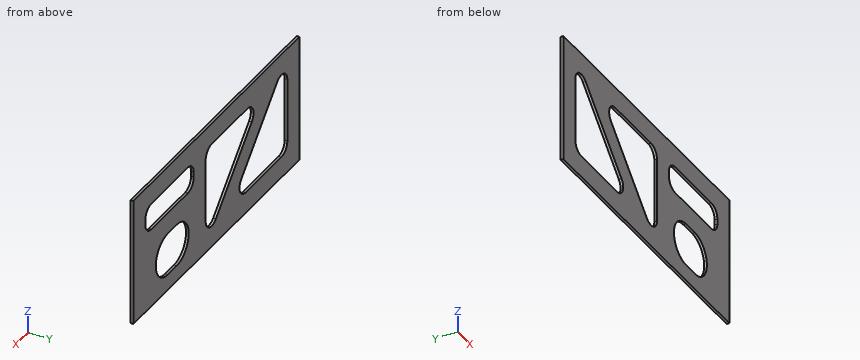
```python
from build123d import *

# Parameters (mm, degrees)
SKETCH1_W           = 352.425
SKETCH1_H           = 152.4
BOSS_EXTRUDE1_DEPTH = 1.5875
CUT_EXTRUDE1_DEPTH  = 4.175


with BuildPart() as part:
    # Sketch1 → Boss-Extrude1 (new body, symmetric)
    with BuildSketch(Plane(origin=(0, 0, 0), x_dir=(1, 0, 0), z_dir=(0, 1, 0))):
        Rectangle(SKETCH1_W, SKETCH1_H)
    extrude(amount=BOSS_EXTRUDE1_DEPTH, both=True)

    # Sketch2 → Cut-Extrude1 (cut, through all)
    with BuildSketch(Plane(origin=(0, 1.5875, 0), x_dir=(1, 0, 0), z_dir=(0, 1, 0))):
        with BuildLine():
            Line((103.1875, 6.35), (84.1375, 6.35))
            ThreePointArc((84.1375, 6.35), (58.7375, 31.75), (84.1375, 57.15))
            Line((84.1375, 57.15), (103.1875, 57.15))
            ThreePointArc((103.1875, 57.15), (128.5875, 31.75), (103.1875, 6.35))
        make_face()
        with BuildLine():
            Line((-138.1125, 50.8), (-61.9125, 50.8))
            ThreePointArc((-61.9125, 50.8), (-50.179229937, 42.960079591), (-52.932243879, 29.119743879))
            Line((-52.932243879, 29.119743879), (-129.132243879, -47.080256121))
            ThreePointArc((-129.132243879, -47.080256121), (-142.972579591, -49.833270063), (-150.8125, -38.1))
            Line((-150.8125, -38.1), (-150.8125, 38.1))
            ThreePointArc((-150.8125, 38.1), (-147.092756121, 47.080256121), (-138.1125, 50.8))
        make_face()
        with BuildLine():
            Line((-66.270451031, -50.8), (9.929548969, -50.8))
            ThreePointArc((9.929548969, -50.8), (18.90980509, -47.080256121), (22.629548969, -38.1))
            Line((22.629548969, -38.1), (22.629548969, 38.1))
            ThreePointArc((22.629548969, 38.1), (14.78962856, 49.833270063), (0.949292847, 47.080256121))
            Line((0.949292847, 47.080256121), (-75.250707153, -29.119743879))
            ThreePointArc((-75.250707153, -29.119743879), (-78.003721094, -42.960079591), (-66.270451031, -50.8))
        make_face()
        with BuildLine():
            Line((60.729548969, -50.8), (138.1125, -50.8))
            ThreePointArc((138.1125, -50.8), (147.092756121, -47.080256121), (150.8125, -38.1))
            Line((150.8125, -38.1), (150.8125, -31.75))
            ThreePointArc((150.8125, -31.75), (147.092756121, -22.769743879), (138.1125, -19.05))
            Line((138.1125, -19.05), (60.729548969, -19.05))
            ThreePointArc((60.729548969, -19.05), (51.749292847, -22.769743879), (48.029548969, -31.75))
            Line((48.029548969, -31.75), (48.029548969, -38.1))
            ThreePointArc((48.029548969, -38.1), (51.749292847, -47.080256121), (60.729548969, -50.8))
        make_face()
    extrude(amount=-CUT_EXTRUDE1_DEPTH, mode=Mode.SUBTRACT)


solid = part.part
```
The model under review builds one solid part; all positions refer to its coordinate system, in mm. Give positions to 0.01 mm unless a question says otherwise; leave off trailing zeros. Write each loop counter-clockwise with the first axis right and the second up, starting at its lowest first coordinate (ties: lowest second). Pieces come first, ordered by that corner, then holes. Notation, with made-up numbers: M 63.5,-7.75 L 111.5,-7.75 A17 ccw 111.5,25.25 Z; hole C 87,-29.75 d5. An arc over 180 degrees is marked long. Answer in a Markdown table with one row per item.
Item 1: For line 1 along Z through (x, y) = (97, -1); line 2 along X through (y, z) = (1.25, 9.5); line 3 along X through (y, z) = (-0.7, 3.5), list the stretches that pass through material, from the lowest coordinate up.
Check sheet entries:
| item | result |
|---|---|
| line 1 | -76.2 to -57.15, -6.35 to 19.05, 50.8 to 76.2 |
| line 2 | -176.21 to -150.81, -91.55 to -55.63, 22.63 to 176.21 |
| line 3 | -176.21 to -150.81, -85.55 to -49.63, 22.63 to 176.21 |
Item 2: Add section A-A on y = -0.75. Give the boundary of the cut face in (x, z), plus the area to 3 significant figures.
Check sheet entries:
| item | result |
|---|---|
| outline | M -176.21,-76.2 L 176.21,-76.2 L 176.21,76.2 L -176.21,76.2 Z; hole M -150.81,-38.1 A12.7 ccw -138.11,-50.8 L -61.91,-50.8 A12.7 ccw -52.93,-29.12 L -129.13,47.08 A12.7 ccw -150.81,38.1 Z; hole M -75.25,29.12 L 0.95,-47.08 A12.7 ccw 22.63,-38.1 L 22.63,38.1 A12.7 ccw 9.93,50.8 L -66.27,50.8 A12.7 ccw Z; hole M 48.03,31.75 A12.7 ccw 60.73,19.05 L 138.11,19.05 A12.7 ccw 150.81,31.75 L 150.81,38.1 A12.7 ccw 138.11,50.8 L 60.73,50.8 A12.7 ccw 48.03,38.1 Z; hole M 84.14,-57.15 L 103.19,-57.15 A25.4 ccw 103.19,-6.35 L 84.14,-6.35 A25.4 ccw Z |
| area | 34,200 mm2 |
Item 3: Add section C-C on x = -112. Give the boundary of the cut face in (y, z).
Check sheet entries:
| item | result |
|---|---|
| outline | M -1.59,-76.2 L 1.59,-76.2 L 1.59,-50.8 L -1.59,-50.8 Z; M -1.59,29.95 L 1.59,29.95 L 1.59,76.2 L -1.59,76.2 Z |
Item 4: Add section B-B on x = 92. Give the boundary of the cut face in (y, z).
Check sheet entries:
| item | result |
|---|---|
| outline | M -1.59,-76.2 L 1.59,-76.2 L 1.59,-57.15 L -1.59,-57.15 Z; M -1.59,-6.35 L 1.59,-6.35 L 1.59,19.05 L -1.59,19.05 Z; M -1.59,50.8 L 1.59,50.8 L 1.59,76.2 L -1.59,76.2 Z |
